from build123d import *

# Parameters (mm, degrees)
SKETCH_1_R      = 1.5
EXTRUDE_1_DEPTH = 25
EXTRUDE_START   = 15
SKETCH_2_R      = 2
SKETCH_2_R_2    = 1.5
EXTRUDE_2_DEPTH = 15
SKETCH_3_R      = 1.5
EXTRUDE_3_DEPTH = 3


with BuildPart() as part:
    # 草图1 → 凸台-拉伸1 (new body)
    with BuildSketch(Plane(origin=(0, 0, 0), x_dir=(1, 0, 0), z_dir=(0, 1, 0))):
        with Locations(Location((0, 0, 0), (0, 0, 270))):
            Circle(SKETCH_1_R)
    extrude(amount=EXTRUDE_1_DEPTH)

    # 草图2 → 凸台-拉伸2 (add)
    with BuildSketch(Plane(origin=(0, 18, 0), x_dir=(-1, 0, 0), z_dir=(0, -1, 0)).offset(EXTRUDE_START)):
        with Locations(Location((0, 0, 0), (0, 0, 90))):
            Circle(SKETCH_2_R)
        with Locations(Location((0, 0, 0), (0, 0, 90))):
            Circle(SKETCH_2_R_2, mode=Mode.SUBTRACT)
    extrude(amount=-EXTRUDE_2_DEPTH)

    # 草图3 → 凸台-拉伸3 (add)
    with BuildSketch(Plane(origin=(0, 18, 0), x_dir=(1, 0, 0), z_dir=(0, 1, 0))):
        with BuildLine():
            Line((0.91625301, 1.777774007), (-1.022249701, 1.719012958))
            ThreePointArc((-1.022249701, 1.719012958), (0.060597358, -1.999081779), (0.91625301, 1.777774007))
        make_face()
        with Locations(Location((0, 0, 0), (0, 0, 90))):
            Circle(SKETCH_3_R, mode=Mode.SUBTRACT)
    extrude(amount=EXTRUDE_3_DEPTH)


solid = part.part
Could you check a few things on this model? Use its own coordinates, in mm. A direction names the side the tool comes from. Round coordinates to 2 decimals unless told otherwise and drop trailing zeros. Write each loop counter-clockwise with the first axis right and the second up, starting at its lowest first coordinate (ties: lowest second). Pieces come first, ordered by that corner, then holes. Notation, with made-up numbers: (25, -2) - (44, -2) arc R21 cw to (44, 37) - close; hole circle Ø6 at (2, -39). An arc over 180 degrees is marked (long way). Put each result on its own line as item: value. Start each with the question number.
(1) For faces 1 (the cylindrical face through (0.45, 22.97, 1.43)), 2 (the flat face through (0, 25, 0)), 3 (the cylindrical face through (0.45, 1.48, 1.43)), which set-ups out of +Z, -Z, +X, -X, +Y, -Y let a thin tool reach every point of the face, with its end or its side?
(2) I need wall thicknesses on probe 1 along Y at (x, z) = (0.9, -1.5); probe 2 along Z at (x, y) = (0.95, 16.5); probe 3 along Z at (x, y) = (-1.3, 19.75). Which ranges of each line are inside material? Lowest first, please.
(3) I want a section at C-C, the plane y = 11. Please give me the cut outline in (x, z).
(4) I want a section at B-B, the plane z = 0. Please give me the cut outline in (x, y).
(5) I want a section at A-A, the plane x = 0. Please give me the cut outline in (y, z).
(6) I want a section at D-D, the plane x = 1.2. Please give me the cut outline in (y, z).
(7) Will this pin go through, and if not, where does the flat tip stop? pin 1 (2 mm diameter, centred on x = 1, y = 19.5, fed in from -Z).
Here are the results:
1. face 1: +Y
1. face 2: +Z, -Z, +X, -X, +Y
1. face 3: -Y
2. probe 1: y = 3 to 21
2. probe 2: z = -1.76 to 1.76
2. probe 3: z = -1.52 to 1.52
3. outline: circle Ø4 at (0, 0)
4. outline: (-2, 3) - (-1.5, 3) - (-1.5, 0) - (1.5, 0) - (1.5, 3) - (2, 3) - (2, 21) - (1.5, 21) - (1.5, 25) - (-1.5, 25) - (-1.5, 21) - (-2, 21) - close
5. outline: (0, -1.5) - (3, -1.5) - (3, -2) - (18, -2) - (18, -1.75) - (21, -1.75) - (21, -1.5) - (25, -1.5) - (25, 1.5) - (21, 1.5) - (21, 2) - (3, 2) - (3, 1.5) - (0, 1.5) - close
6. outline: (0, -0.9) - (3, -0.9) - (3, -1.6) - (21, -1.6) - (21, -0.9) - (25, -0.9) - (25, 0.9) - (21, 0.9) - (21, 1.6) - (3, 1.6) - (3, 0.9) - (0, 0.9) - close
7. pin 1: stops at z = -1.78
